Source: CAD feature listing. Evaluate the final solid. Frame: model axes, mm. Round coordinates to 2 decimals unless told otherwise and drop trailing zeros. Order: outer loops, then holes, each group sorted by start corner. A loop starts at its lowest first (then second) coordinate and runs counter-clockwise, first axis right, second up. Notation, with made-up numbers: (54.25, -35.75) -> (102.25, -35.75) arc R21 cw to (102.25, -5.75) -> close; hole circle Ø3 at (-22.75, 68). An arc over 180 degrees is marked (long way). Write item = value, one per line. Start each with the question number.
(1) Ray query, line 1 (Y direction, x = 0, z = -11); line 2 (Y direction, x = 4.25, z = 14); line 3 (X direction, y = -0.5, z = -12). Return the intervals inside material, ascending.
(2) Cut plane A-A on y = 0. Return the cut outline in (x, z).
(3) Contact query for flat-ended pins moving along their axis: pin 1 Ø1 at (x, z) = (0, 1) entering from -Y; pin 2 Ø1.6 at (x, z) = (-0.5, 0) entering from +Y. Output: stop coordinate, or through.
from build123d import *

# Parameters (mm, degrees)
F0_R     = 1.25
F1_DEPTH = 20


with BuildPart() as f1:
    # F0 (on Top) → F1 (new body, symmetric)
    with BuildSketch(Plane.XY):
        with BuildLine():
            Line((-2, 1), (-2, 0))
            Line((-2, 0), (-2, -1))
            Line((-2, -1), (-3.646791, -2.962569))
            ThreePointArc((-3.646791, -2.962569), (-3.868404, -3.02195), (-4, -2.834012))
            Line((-4, -2.834012), (-4, -1.7))
            ThreePointArc((-4, -1.7), (-4.058579, -1.558579), (-4.2, -1.5))
            Line((-4.2, -1.5), (-4.8, -1.5))
            ThreePointArc((-4.8, -1.5), (-4.941421, -1.558579), (-5, -1.7))
            Line((-5, -1.7), (-5, -4.8))
            ThreePointArc((-5, -4.8), (-4.984776, -4.876537), (-4.941421, -4.941421))
            ThreePointArc((-4.941421, -4.941421), (-4.876537, -4.984776), (-4.8, -5))
            Line((-4.8, -5), (-1.7, -5))
            ThreePointArc((-1.7, -5), (-1.558579, -4.941421), (-1.5, -4.8))
            Line((-1.5, -4.8), (-1.5, -4.2))
            ThreePointArc((-1.5, -4.2), (-1.558579, -4.058579), (-1.7, -4))
            Line((-1.7, -4), (-2.834012, -4))
            ThreePointArc((-2.834012, -4), (-3.02195, -3.868404), (-2.962569, -3.646791))
            Line((-2.962569, -3.646791), (-1, -2))
            Line((-1, -2), (0, -2))
            Line((0, -2), (1, -2))
            Line((1, -2), (2.962569, -3.646791))
            ThreePointArc((2.962569, -3.646791), (3.02195, -3.868404), (2.834012, -4))
            Line((2.834012, -4), (1.7, -4))
            ThreePointArc((1.7, -4), (1.558579, -4.058579), (1.5, -4.2))
            Line((1.5, -4.2), (1.5, -4.8))
            ThreePointArc((1.5, -4.8), (1.558579, -4.941421), (1.7, -5))
            Line((1.7, -5), (4.8, -5))
            ThreePointArc((4.8, -5), (4.876537, -4.984776), (4.941421, -4.941421))
            ThreePointArc((4.941421, -4.941421), (4.984776, -4.876537), (5, -4.8))
            Line((5, -4.8), (5, -1.7))
            ThreePointArc((5, -1.7), (4.941421, -1.558579), (4.8, -1.5))
            Line((4.8, -1.5), (4.2, -1.5))
            ThreePointArc((4.2, -1.5), (4.058579, -1.558579), (4, -1.7))
            Line((4, -1.7), (4, -2.834012))
            ThreePointArc((4, -2.834012), (3.868404, -3.02195), (3.646791, -2.962569))
            Line((3.646791, -2.962569), (2, -1))
            Line((2, -1), (2, 0))
            Line((2, 0), (2, 1))
            Line((2, 1), (3.646791, 2.962569))
            ThreePointArc((3.646791, 2.962569), (3.868404, 3.02195), (4, 2.834012))
            Line((4, 2.834012), (4, 1.7))
            ThreePointArc((4, 1.7), (4.058579, 1.558579), (4.2, 1.5))
            Line((4.2, 1.5), (4.8, 1.5))
            ThreePointArc((4.8, 1.5), (4.941421, 1.558579), (5, 1.7))
            Line((5, 1.7), (5, 4.8))
            ThreePointArc((5, 4.8), (4.984776, 4.876537), (4.941421, 4.941421))
            ThreePointArc((4.941421, 4.941421), (4.876537, 4.984776), (4.8, 5))
            Line((4.8, 5), (1.7, 5))
            ThreePointArc((1.7, 5), (1.558579, 4.941421), (1.5, 4.8))
            Line((1.5, 4.8), (1.5, 4.2))
            ThreePointArc((1.5, 4.2), (1.558579, 4.058579), (1.7, 4))
            Line((1.7, 4), (2.834012, 4))
            ThreePointArc((2.834012, 4), (3.02195, 3.868404), (2.962569, 3.646791))
            Line((2.962569, 3.646791), (1, 2))
            Line((1, 2), (0, 2))
            Line((0, 2), (-1, 2))
            Line((-1, 2), (-2.962569, 3.646791))
            ThreePointArc((-2.962569, 3.646791), (-3.02195, 3.868404), (-2.834012, 4))
            Line((-2.834012, 4), (-1.7, 4))
            ThreePointArc((-1.7, 4), (-1.558579, 4.058579), (-1.5, 4.2))
            Line((-1.5, 4.2), (-1.5, 4.8))
            ThreePointArc((-1.5, 4.8), (-1.558579, 4.941421), (-1.7, 5))
            Line((-1.7, 5), (-4.8, 5))
            ThreePointArc((-4.8, 5), (-4.876537, 4.984776), (-4.941421, 4.941421))
            ThreePointArc((-4.941421, 4.941421), (-4.984776, 4.876537), (-5, 4.8))
            Line((-5, 4.8), (-5, 1.7))
            ThreePointArc((-5, 1.7), (-4.941421, 1.558579), (-4.8, 1.5))
            Line((-4.8, 1.5), (-4.2, 1.5))
            ThreePointArc((-4.2, 1.5), (-4.058579, 1.558579), (-4, 1.7))
            Line((-4, 1.7), (-4, 2.834012))
            ThreePointArc((-4, 2.834012), (-3.868404, 3.02195), (-3.646791, 2.962569))
            Line((-3.646791, 2.962569), (-2, 1))
        make_face()
        Circle(F0_R, mode=Mode.SUBTRACT)
    extrude(amount=F1_DEPTH, both=True)


solid = f1.part
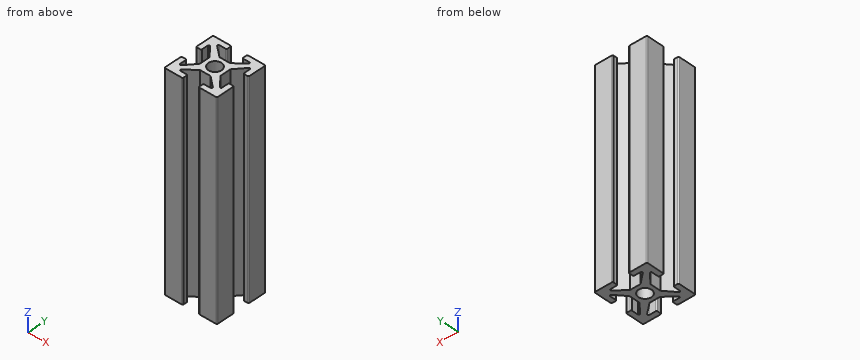
Evaluation:
q1.line_1 = -2 to -1.25, 1.25 to 2
q1.line_2 = -5 to -1.5, 1.5 to 5
q1.line_3 = -2 to -1.15, 1.15 to 2
q2.outline = (-2, -20) -> (-1.25, -20) -> (-1.25, 20) -> (-2, 20) -> close; (1.25, -20) -> (2, -20) -> (2, 20) -> (1.25, 20) -> close
q3.pin_1 = -2
q3.pin_2 = 2.25
